from build123d import *

# Parameters (mm, degrees)
F0_R     = 7
F0_R_2   = 1.5
F1_DEPTH = 3
F2_R     = 1.551902
F3_DEPTH = 1.5
F4_W     = 0.3
F4_H     = 6
F5_DEPTH = 6
F6_R     = 2
F7_R     = 1.5
F8_DEPTH = 4


with BuildPart() as f1:
    # F0 (on Top) → F1 (new body)
    with BuildSketch(Plane.XY):
        Circle(F0_R)
        Circle(F0_R_2, mode=Mode.SUBTRACT)
    extrude(amount=F1_DEPTH)

    # F2 (on face) → F3 (join)
    with BuildSketch(Plane(origin=(0, 0, 0), x_dir=(1, 0, 0), z_dir=(0, 0, -1))):
        Circle(F2_R)
    extrude(amount=-F3_DEPTH)

    # F4 (on face) → F5 (join)
    with BuildSketch(Plane(origin=(0, 0, 0), x_dir=(1, 0, 0), z_dir=(0, 0, -1))):
        with Locations((-3.15, 0)):
            Rectangle(F4_W, F4_H)
        with Locations((3.15, 0)):
            Rectangle(F4_W, F4_H)
    extrude(amount=F5_DEPTH)

    # F6
    f6_edges = [f1.edges().sort_by_distance(p)[0] for p in [
        (-3.15, -3, -6),
        (-3.15, 3, -6),
        (3.15, 3, -6),
        (3.15, -3, -6),
    ]]
    fillet(f6_edges, radius=F6_R)

    # F7 (on face) → F8 (join)
    with BuildSketch(Plane(origin=(0, 0, 0), x_dir=(1, 0, 0), z_dir=(0, 0, -1))):
        Circle(F7_R)
    extrude(amount=-F8_DEPTH)


solid = f1.part
The listing builds one solid part. Answer for the finished solid, in the listing's coordinates (mm). A direction names the side the tool comes from. Coordinates: 2 decimals unless noted, no trailing zeros. Write each loop counter-clockwise with the first axis right and the second up, starting at its lowest first coordinate (ties: lowest second). Pieces come first, ordered by that corner, then holes. Notation, with made-up numbers: (61.5, 84) -> (69.5, 84) arc R8 cw to (69.5, 90) -> close; hole circle Ø8 at (5, -37). An arc over 180 degrees is marked (long way). One line per question, with ' | ' between items.
1. Section C-C (x = 0) is taken. Determine the outline of the cut face in (y, z), and give its area (3 significant figures).
Verdict:
outline: (-7, 0) -> (7, 0) -> (7, 3) -> (1.5, 3) -> (1.5, 4) -> (-1.5, 4) -> (-1.5, 3) -> (-7, 3) -> close | area: 45.0 mm^2
2. Section B-B (y = 0) is taken. Determine the outline of the cut face in (x, z), and give its area (3 significant figures).
Verdict:
outline: (-7, 0) -> (-3.3, 0) -> (-3.3, -6) -> (-3, -6) -> (-3, 0) -> (3, 0) -> (3, -6) -> (3.3, -6) -> (3.3, 0) -> (7, 0) -> (7, 3) -> (1.5, 3) -> (1.5, 4) -> (-1.5, 4) -> (-1.5, 3) -> (-7, 3) -> close | area: 48.6 mm^2
3. Given pin 1 Ø1.8 at (y, z) = (0, -4) entering from +X; pin 2 Ø8 at (x, y) = (-0.5, -4) entering from +Z; pin 3 Ø4 at (x, y) = (3.5, 1) entering from +Z; pin 4 Ø5 at (y, z) = (4, -4.5) entering from -X, each flat-ended and moving along its own axis, determine where each tip first touches the part or whether it passes through.
Verdict:
pin 1: stops at x = 3.3 | pin 2: stops at z = 4 | pin 3: stops at z = 3 | pin 4: stops at x = -3.3
4. Which of the six approach directions +Z, -Z, +X, -X, +Y, -Y give full straight-line access (tool end or side, diameter ignored) to faces 1 (the flat face through (-3.3, 0, -3)), 2 (the flat face through (-3, 0, -3)), 3 (the cylindrical face through (-1.5, -0.07, 3.49))?
Verdict:
face 1: -Z, -X, +Y, -Y | face 2: -Z, +Y, -Y | face 3: +Z
5. Straight lines are drawn through the part: line 1 (X direction, y = -0.75, z = -2.5); line 2 (Z direction, x = 4.5, y = -0.75); line 3 (Z direction, x = -1.25, y = -0.5). For each, find the intervals that lie inside material, in ascending order.
Verdict:
line 1: x = -3.3 to -3, 3 to 3.3 | line 2: z = 0 to 3 | line 3: z = 0 to 4
6. For a pull along X with two mould halves and no side action, classify faces 4 (the flat face through (0, 2, 3)), 5 (the flat face through (3, 0, -3)), 6 (the flat face through (3.3, 0, -3)) as released by +X, released by -X, zero draft, split by the parting line, or undercut.
Verdict:
face 4: zero draft | face 5: undercut | face 6: released by +X
7. Section A-A (z = -1.5) is taken. Determine the outline of the cut face in (x, y), and give its area (3 significant figures).
Verdict:
outline: (-3.3, -3) -> (-3, -3) -> (-3, 3) -> (-3.3, 3) -> close; (3, -3) -> (3.3, -3) -> (3.3, 3) -> (3, 3) -> close | area: 3.60 mm^2
8. Section D-D (z = 1.5) is taken. Determine the outline of the cut face in (x, y), and give its area (3 significant figures).
Verdict:
outline: circle Ø14 at (0, 0) | area: 154 mm^2
